Autodesk Inventor part; units mm, degrees
ref_plane "YZ Plane" through (0, 0, 0) normal (1, 0, 0) x (0, 1, 0)
ref_plane "XZ Plane" through (0, 0, 0) normal (0, 1, 0) x (-1, 0, 0)
ref_plane "XY Plane" through (0, 0, 0) normal (0, 0, 1) x (1, 0, 0)
sketch "Sketch3" plane through (0, 0, 0) normal (0, 1, 0) x (-1, 0, 0)
  line L0 (0, 0) -> (29, 0)
  line L1 (29, 0) -> (29, -29)
  line L2 (29, -29) -> (0, -29)
  line L3 (0, -29) -> (0, 0)
  dimension "d8" = 29
  dimension "d9" = 29
extrude "Extrusion3" add sketch "Sketch3" along normal blind 2
sketch "Sketch4" plane through (0, 2, 0) normal (0, 1, 0) x (1, 0, 0)
  line L0 (-29, 29) -> (-29, 0)
  line L1 (-29, 0) -> (0, 0)
  line L2 (0, 0) -> (0, 29)
  line L3 (0, 29) -> (-29, 29)
  line L4 (-27, 2) -> (-27, 27)
  line L5 (-27, 27) -> (-2, 27)
  line L6 (-2, 27) -> (-2, 2)
  line L7 (-2, 2) -> (-27, 2)
  line L8 (-25, 25) -> (-25, 4)
  line L9 (-25, 4) -> (-4, 4)
  line L10 (-4, 4) -> (-4, 25)
  line L11 (-4, 25) -> (-25, 25)
  dimension "d12" = 2
  dimension "d13" = 2
extrude "Extrusion4" add sketch "Sketch4" along normal blind 2 contours L4 L5 L6 L7
sketch "Sketch5" plane through (0, 0, 0) normal (0, -1, 0) x (1, 0, 0)
  line L0 (-4, -4) -> (-4, -25)
  line L1 (-4, -25) -> (-25, -25)
  line L2 (-25, -25) -> (-25, -4)
  line L3 (-25, -4) -> (-4, -4)
  line L4 (-4, -4) -> (-7, -4)
  line L5 (-7, -4) -> (-7, -7)
  line L6 (-7, -7) -> (-4, -7)
  line L7 (-4, -7) -> (-4, -4)
  point P0 (0, 0)
  dimension "d16" = 3
  dimension "d17" = 3
hole "Hole1" at (-7, 0, -7) direction (0, 1, 0) diameter 4 end through all
properties part number "waterBallonHolderCapv2"
Geometry check sheet. Reference: the model listing, model coordinates, mm. A direction names the side the tool comes from. Round coordinates to 2 decimals unless told otherwise and drop trailing zeros. Loops run counter-clockwise (first coordinate to the right, second up) from the corner with the lowest first, then second, coordinate; pieces in that order, holes last. Notation, with made-up numbers: (10.5, -13.5) - (58.5, -13.5) arc R24 cw to (58.5, 25.5) - close; hole circle Ø5 at (38.25, -37.5). An arc over 180 degrees is marked (long way). Answer as CSV lines item,"result".
(1) Depth check by flat-ended pin: pin 1 Ø0.6 at (y, z) = (2.5, -13) entering from -X; pin 2 Ø1.6 at (x, y) = (-13.5, 3) entering from -Z; pin 3 Ø1 at (x, y) = (-19, 3) entering from +Z. Enter the tip coordinate at first touch or a pass-through.
Output values:
pin 1,"stops at x = -27"
pin 2,"stops at z = -27"
pin 3,"stops at z = -2"
(2) Cross-section at A-A, the plane x = -7. Enter the section's corners in (y, z).
Output values:
outline,"(0, -29) - (2, -29) - (2, -27) - (4, -27) - (4, -25) - (2, -25) - (2, -9) - (0, -9) - close; (0, -5) - (2, -5) - (2, -4) - (4, -4) - (4, -2) - (2, -2) - (2, 0) - (0, 0) - close"
(3) Cross-section at B-B, the plane z = -7. Enter the section's corners in (x, y), and give its area (3 significant figures).
Output values:
outline,"(-29, 0) - (-9, 0) - (-9, 2) - (-25, 2) - (-25, 4) - (-27, 4) - (-27, 2) - (-29, 2) - close; (-5, 0) - (0, 0) - (0, 2) - (-2, 2) - (-2, 4) - (-4, 4) - (-4, 2) - (-5, 2) - close"
area,"58.0 mm²"
(4) Release check for a two-part mould opening along X. For faces 6 (the face through (-4, 3, -14)), 7 (the face through (-1, 2, -14)), 8 (the face through (-27, 3, -14)), 9 (the face through (-14, 3, -25)) record: released by +X, released by -X, zero draft, split by the parting line, or undercut.
Output values:
face 6,"undercut"
face 7,"zero draft"
face 8,"released by -X"
face 9,"undercut"
(5) Material ranges on line 1 along Z through (x, y) = (-13.25, 3.4); line 2 along X through (y, z) = (0.8, -7), recorded low to high.
Output values:
line 1,"z = -27 to -25, -4 to -2"
line 2,"x = -29 to -9, -5 to 0"
(6) Set-up check for faces 1 (the face through (-15, 3, -4)), 2 (the face through (-2, 3, -15)), 3 (the face through (-15, 3, -27)), 4 (the face through (-8.352, 1.014, -5.526)), 5 (the face through (-14, 3, -2)): record each of +Z, -Z, +X, -X, +Y, -Y from which the full face is reachable in a straight line by a thin tool's end or side.
Output values:
face 1,"+Y"
face 2,"+Z, -Z, +X, +Y"
face 3,"-Z, +X, -X, +Y"
face 4,"+Y, -Y"
face 5,"+Z, +X, -X, +Y"
(7) Cross-section at D-D, the plane x = -25.5. Enter the section's corners in (y, z), and give its area (3 significant figures).
Output values:
outline,"(0, -29) - (2, -29) - (2, -27) - (4, -27) - (4, -2) - (2, -2) - (2, 0) - (0, 0) - close"
area,"108 mm²"
(8) Cross-section at C-C, the plane y = 2.4. Enter the section's corners in (x, z), and give its area (3 significant figures).
Output values:
outline,"(-27, -27) - (-2, -27) - (-2, -2) - (-27, -2) - close; hole (-25, -25) - (-4, -25) - (-4, -4) - (-25, -4) - close"
area,"184 mm²"
